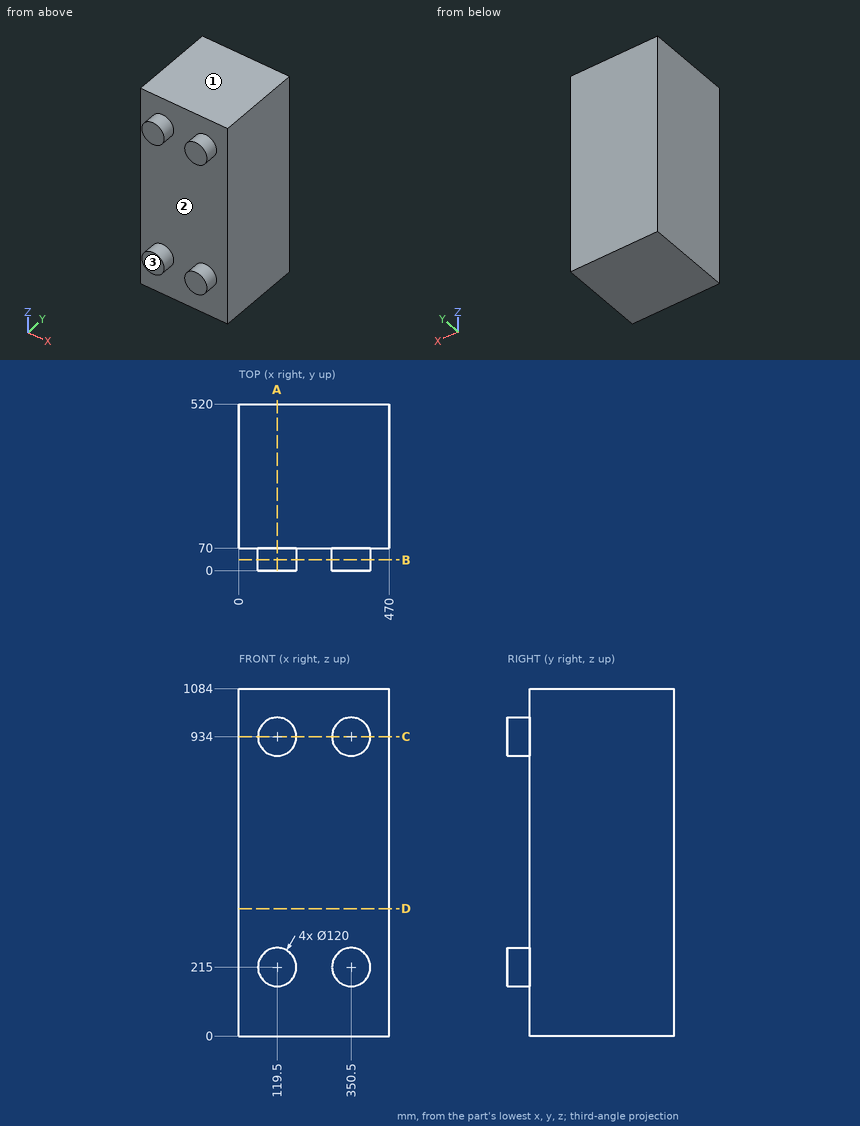
Design review of the part shown in the three views and the two pictorial views. Dimensions are in mm from the part's minimum x, y and z. Give positions to 0.01 mm unless a question says otherwise; leave off trailing zeros. Write each loop counter-clockwise with the first axis right and the second up, starting at its lowest first coordinate (ties: lowest second). Pieces come first, ordered by that corner, then holes.
Item 1: Take a section at B-B (y = 33.5). Give the boundary of the cut face in (x, z).
Item 2: The part is to be moulded in two halves that separate along Z. For the marked faces 1, 2 and 3, say which applies: +Z half, -Z half, draft (parallel to the pull), parting line (faces both ways), or undercut.
Item 3: Wall thickness on probe 1 along Y at (x, z) = (444.5, 899.5); probe 2 along Z at (x, y) = (367, 28.5); probe 3 along Z at (x, y) = (147, 24): over which ranges is each line inside the solid? List them lowest first.
Item 4: Take a section at A-A (x = 119.5). Give the boundary of the cut face in (y, z).
Item 5: Take a section at C-C (z = 934). Give the boundary of the cut face in (x, y), and give its area (3 significant figures).
Item 6: Take a section at D-D (z = 397.5). Give the boundary of the cut face in (x, y).
Established:
1. outline: circle Ø120 at (119.5, 215); circle Ø120 at (119.5, 934); circle Ø120 at (350.5, 215); circle Ø120 at (350.5, 934)
2. face 1: +Z half
2. face 2: undercut
2. face 3: draft
3. probe 1: y = 70 to 520
3. probe 2: z = 157.31 to 272.69, 876.31 to 991.69
3. probe 3: z = 161.67 to 268.33, 880.67 to 987.33
4. outline: (0, 155) - (70, 155) - (70, 0) - (520, 0) - (520, 1084) - (70, 1084) - (70, 994) - (0, 994) - (0, 874) - (70, 874) - (70, 275) - (0, 275) - close
5. outline: (0, 70) - (59.5, 70) - (59.5, 0) - (179.5, 0) - (179.5, 70) - (290.5, 70) - (290.5, 0) - (410.5, 0) - (410.5, 70) - (470, 70) - (470, 520) - (0, 520) - close
5. area: 228,000 mm2
6. outline: (0, 70) - (470, 70) - (470, 520) - (0, 520) - close
